Read the model definition and answer for the solid it produces. Units are mm, in the model's axes. A direction names the side the tool comes from. Give positions to 0.01 mm unless a question says otherwise; leave off trailing zeros. Order: outer loops, then holes, each group sorted by start corner. A loop starts at its lowest first (then second) coordinate and runs counter-clockwise, first axis right, second up. Notation, with made-up numbers: (-37, -29.75) - (-19, -29.75) arc R22 ccw to (-19, 2.25) - close; hole circle Ø7 at (10.25, 37). An arc over 180 degrees is marked (long way). Return JSON: item names as keys, results as strings.
```python
from build123d import *

# Parameters (mm, degrees)
EXTRUDE_1_DEPTH     = 125.6
EXTRUDE_START       = 1
SKETCH_2_R          = 2
EXTRUDE_2_DEPTH     = 1
SKETCH_3_R          = 2
SKETCH_3_R_2        = 6.5
SKETCH_3_R_3        = 5
EXTRUDE_3_DEPTH     = 1
SKETCH_4_W          = 30
SKETCH_4_H          = 50
CUT_EXTRUDE_1_DEPTH = 20
CUT_EXTRUDE_2_REACH = 174.834
SKETCH_5_W          = 20
SKETCH_5_H          = 2
EXTRUDE_START_2     = -23
EXTRUDE_4_DEPTH     = 10


with BuildPart() as part:
    # 草图1 → 凸台-拉伸1 (new body)
    with BuildSketch(Plane(origin=(0, 0, 0), x_dir=(0, 0, -1), z_dir=(1, 0, 0))):
        with BuildLine():
            Line((0, 0), (0, 41))
            ThreePointArc((0, 41), (-6.150757595, 55.849242405), (-21, 62))
            Line((-21, 62), (-100, 62))
            Line((-100, 62), (-100, 61))
            Line((-100, 61), (-21, 61))
            ThreePointArc((-21, 61), (-6.857864376, 55.142135624), (-1, 41))
            Line((-1, 41), (-1, 1))
            Line((-1, 1), (-35, 1))
            Line((-35, 1), (-35, -7))
            Line((-35, -7), (-34, -7))
            Line((-34, -7), (-34, 0))
            Line((-34, 0), (0, 0))
        make_face()
    extrude(amount=EXTRUDE_1_DEPTH)

    # 草图2 → 凸台-拉伸2 (add)
    with BuildSketch(Plane.ZY.offset(EXTRUDE_START)):
        with BuildLine():
            Line((35, 0), (0, 0))
            Line((0, 0), (0, 41))
            ThreePointArc((0, 41), (6.150757595, 55.849242405), (21, 62))
            Line((21, 62), (100, 62))
            Line((100, 62), (100, 16))
            Line((100, 16), (35, 16))
            Line((35, 16), (35, 0))
        make_face()
        with Locations((94, 20)):
            Circle(SKETCH_2_R, mode=Mode.SUBTRACT)
        with Locations((40, 20)):
            Circle(SKETCH_2_R, mode=Mode.SUBTRACT)
    extrude(amount=-EXTRUDE_2_DEPTH)

    # 草图3 → 凸台-拉伸3 (add)
    with BuildSketch(Plane(origin=(125.6, 0, 0), x_dir=(0, 0, -1), z_dir=(1, 0, 0))):
        with BuildLine():
            Line((-35, 16), (-100, 16))
            Line((-100, 16), (-100, 62))
            Line((-100, 62), (-21, 62))
            ThreePointArc((-21, 62), (-6.150757595, 55.849242405), (0, 41))
            Line((0, 41), (0, 0))
            Line((0, 0), (-35, 0))
            Line((-35, 0), (-35, 16))
        make_face()
        with Locations(Location((-94, 20, 0), (0, 0, 180))):
            Circle(SKETCH_3_R, mode=Mode.SUBTRACT)
        with Locations(Location((-40, 20, 0), (0, 0, 180))):
            Circle(SKETCH_3_R, mode=Mode.SUBTRACT)
        with Locations((-13, 45)):
            Circle(SKETCH_3_R_2, mode=Mode.SUBTRACT)
        with Locations((-10, 10)):
            Circle(SKETCH_3_R_3, mode=Mode.SUBTRACT)
    extrude(amount=EXTRUDE_3_DEPTH)

    # 草图4 → 切除-拉伸1 (cut)
    with BuildSketch(Plane(origin=(0, 62, 0), x_dir=(1, 0, 0), z_dir=(0, 1, 0))):
        with Locations((62.8, -25)):
            Rectangle(SKETCH_4_W, SKETCH_4_H)
    extrude(amount=-CUT_EXTRUDE_1_DEPTH, mode=Mode.SUBTRACT)

    # 草图5 → 切除-拉伸2 (cut, up to next)
    with BuildSketch(Plane(origin=(0, 0, 0), x_dir=(-1, 0, 0), z_dir=(0, 0, -1)), mode=Mode.PRIVATE) as cut_extrude_2_sk1:
        with Locations((-106.6, 36)):
            Rectangle(SKETCH_5_W, SKETCH_5_H)
    cut_extrude_2_tool1 = extrude(cut_extrude_2_sk1.sketch, amount=-CUT_EXTRUDE_2_REACH, mode=Mode.PRIVATE) & part.part
    # 草图5 → 切除-拉伸2 (cut, up to next)
    with BuildSketch(Plane(origin=(0, 0, 0), x_dir=(-1, 0, 0), z_dir=(0, 0, -1)), mode=Mode.PRIVATE) as cut_extrude_2_sk2:
        with Locations((-19, 36)):
            Rectangle(SKETCH_5_W, SKETCH_5_H)
    cut_extrude_2_tool2 = extrude(cut_extrude_2_sk2.sketch, amount=-CUT_EXTRUDE_2_REACH, mode=Mode.PRIVATE) & part.part
    add(cut_extrude_2_tool1.solids().sort_by_distance((106.6, 36, 0))[0], mode=Mode.SUBTRACT)
    add(cut_extrude_2_tool2.solids().sort_by_distance((19, 36, 0))[0], mode=Mode.SUBTRACT)

    # 草图6 → 凸台-拉伸4 (add)
    with BuildSketch(Plane(origin=(126.6, 0, 0), x_dir=(0, 0, -1), z_dir=(1, 0, 0)).offset(EXTRUDE_START_2)):
        with BuildLine():
            Line((-10, 16), (0, 16))
            Line((0, 16), (0, 4))
            Line((0, 4), (-10, 4))
            ThreePointArc((-10, 4), (-10.783157153, 4.051330832), (-11.552914271, 4.204445042))
            Line((-11.552914271, 4.204445042), (-11.164685703, 5.653333782))
            ThreePointArc((-11.164685703, 5.653333782), (-5.5, 10), (-11.164685703, 14.346666218))
            Line((-11.164685703, 14.346666218), (-11.552914271, 15.795554958))
            ThreePointArc((-11.552914271, 15.795554958), (-10.783157153, 15.948669168), (-10, 16))
        make_face()
    extrude(amount=-EXTRUDE_4_DEPTH)


solid = part.part
```
Q1. A cutting plane is placed at B-B (z = 40). Write down the section's boundary in (x, y), and give its area (3 significant figures).
Values:
{"outline": "(-1, 16) - (0, 16) - (0, 18) - (-1, 18) - close; (-1, 22) - (0, 22) - (0, 61) - (47.8, 61) - (47.8, 62) - (-1, 62) - close; (77.8, 61) - (125.6, 61) - (125.6, 22) - (126.6, 22) - (126.6, 62) - (77.8, 62) - close; (125.6, 16) - (126.6, 16) - (126.6, 18) - (125.6, 18) - close", "area": "180 mm²"}
Q2. For faces 1 (the flat face through (62, 1, 18)), 2 (the flat face through (77.8, 61, 18)), 3 (the cylindrical face through (126.09, 11.5, 5.23)), 4 (the flat face through (62, -4, 34)), 5 (the cylindrical face through (-0.507, 20.601, 95.908)), determine the directions among +Z, -Z, +X, -X, +Y, -Y from which every point of the face is accessible in a straight line to the end or side of a thin tool.
Values:
{"face 1": "+Z", "face 2": "-Z, +Y", "face 3": "+X", "face 4": "-Z, +X, -X, -Y", "face 5": "+X, -X"}
Q3. A cutting plane is placed at A-A (y = 10). Write down the section's boundary in (x, z).
Values:
{"outline": "(-1, 0) - (126.6, 0) - (126.6, 5) - (125.6, 5) - (125.6, 1) - (103.6, 1) - (103.6, 5.5) - (93.6, 5.5) - (93.6, 1) - (0, 1) - (0, 35) - (-1, 35) - close; (125.6, 15) - (126.6, 15) - (126.6, 35) - (125.6, 35) - close"}
Q4. Given pin 1 (1 mm diameter, centred on x = 73.5, y = 4, fed in from +Z); pin 2 (10 mm diameter, centred on x = 41, y = 54.5, fed in from -Z); pin 3 (10 mm diameter, centred on x = 30, y = 5.5, fed in from +Z), each flat-ended and moving along its own axis, determine where each tip first touches the part or whether it passes through.
Values:
{"pin 1": "stops at z = 1", "pin 2": "stops at z = 1.8", "pin 3": "stops at z = 35"}
Q5. Consider L1, parallel to Z at x = 125.9, y = 20; L2, parallel to X at y = 51.5, z = 87; L3, parallel to Y at x = 117, z = 28. Determine where each line is inside the solid, lowest interval first.
Values:
{"L1": "z = 0 to 38, 42 to 92, 96 to 100", "L2": "x = -1 to 0, 125.6 to 126.6", "L3": "y = 0 to 1, 61 to 62"}
Q6. Determine the mould class of faces 6 (the cylindrical face through (34.01, 55.297, 7.014)), 7 (the cylindrical face through (-0.507, 21.983, 39.74)), 8 (the flat face through (126.6, 38, 49)) for opening direction X: released by +X, released by -X, zero draft, split by the parting line, or undercut.
Values:
{"face 6": "undercut", "face 7": "zero draft", "face 8": "released by +X"}
Q7. A cutting plane is placed at D-D (z = 13). Write down the section's boundary in (x, y), and give its area (3 significant figures).
Values:
{"outline": "(-1, 0) - (126.6, 0) - (126.6, 6) - (125.6, 6) - (125.6, 1) - (0, 1) - (0, 59.33) - (47.8, 59.33) - (47.8, 60.42) - (-1, 60.42) - close; (77.8, 59.33) - (125.6, 59.33) - (125.6, 51.5) - (126.6, 51.5) - (126.6, 60.42) - (77.8, 60.42) - close; (125.6, 14) - (126.6, 14) - (126.6, 38.5) - (125.6, 38.5) - close", "area": "329 mm²"}
Q8. A cutting plane is placed at C-C (x = 73). Write down the section's boundary in (y, z).
Values:
{"outline": "(-7, 34) - (0, 34) - (0, 0) - (41, 0) arc R21 ccw to (42, 0.02) - (42, 1.03) arc R20 cw to (41, 1) - (1, 1) - (1, 35) - (-7, 35) - close; (61, 50) - (62, 50) - (62, 100) - (61, 100) - close"}
